Geometry check sheet. Reference: drawing and pictorial views, mm from the part's lowest x, y, z. A direction names the side the tool comes from. Coordinates: 2 decimals unless noted, no trailing zeros. Loops run counter-clockwise (first coordinate to the right, second up) from the corner with the lowest first, then second, coordinate; pieces in that order, holes last. Notation, with made-up numbers: (58.25, -16.75) - (96.25, -16.75) arc R32 ccw to (96.25, 16.25) - close; hole circle Ø9 at (-23.75, 87.5). An arc over 180 degrees is marked (long way). Use a Markdown table: item, result. Add a question column.
1) Thickness scan on line 1 (X direction, y = 1.25, z = 8.75); line 2 (X direction, y = 4, z = 1.5); line 3 (Y direction, x = 4, z = 5.75). Record the ranges inside material, lowest first.
2) Sectioned sample at B-B, the plane x = 3.66. Enter the section's corners in (y, z).
3) Sectioned sample at D-D, the plane x = 8. Enter the section's corners in (y, z), then the cut area to 3 significant figures.
4) Draft check along X on the marked faces 3, 4 and 5. Enter one of: pulls with the +X half, pulls with the -X half, needs draft (parallel to the pull), parting line crosses it, or undercut.
5) Sectioned sample at C-C, the plane y = 0.5. Enter the section's corners in (x, z).
6) Tool access check on the marked faces 1 and 2. Record the directions out of +Z, -Z, +X, -X, +Y, -Y that give a thin tool (end or side, any length) a straight path to the whole face; none if there is none.
7) Sectioned sample at A-A, the plane z = 5.5. State how many separate pieces and enclosed holes the cut face has, then the cut area to 3 significant figures.
8) Go/stop test with flat-tipped pins: P1, Ø2, axis at x = 3, z = 1, coming from the +Y side; P2, Ø1, axis at x = 9.5, y = 2, coming from the -Z side. Record where each tip stops, or that it passes through.
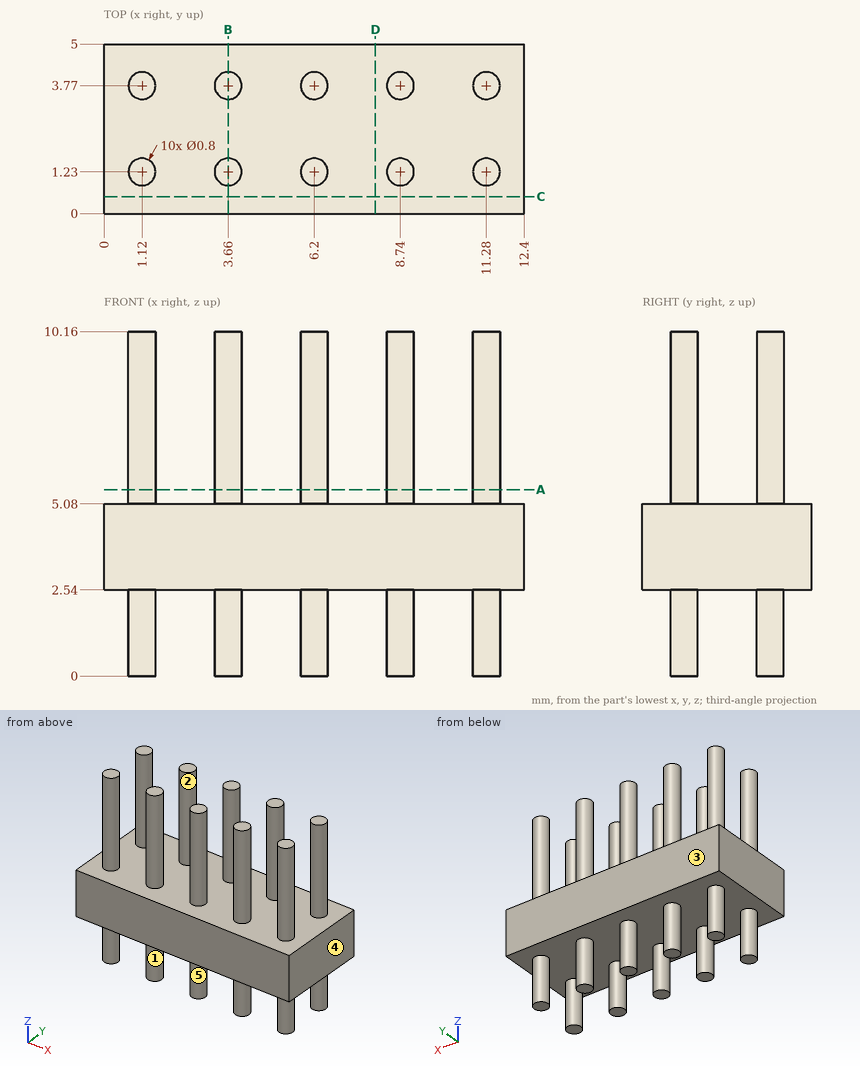
Solved:
| question | item | result |
|---|---|---|
| 1 | line 1 | x = 0.72 to 1.52, 3.26 to 4.06, 5.8 to 6.6, 8.34 to 9.14, 10.88 to 11.68 |
| 1 | line 2 | x = 0.79 to 1.45, 3.33 to 3.99, 5.87 to 6.53, 8.41 to 9.07, 10.95 to 11.61 |
| 1 | line 3 | y = 1.02 to 1.44, 3.56 to 3.98 |
| 2 | outline | (0, 2.54) - (0.83, 2.54) - (0.83, 0) - (1.63, 0) - (1.63, 2.54) - (3.37, 2.54) - (3.37, 0) - (4.17, 0) - (4.17, 2.54) - (5, 2.54) - (5, 5.08) - (4.17, 5.08) - (4.17, 10.16) - (3.37, 10.16) - (3.37, 5.08) - (1.63, 5.08) - (1.63, 10.16) - (0.83, 10.16) - (0.83, 5.08) - (0, 5.08) - close |
| 3 | outline | (0, 2.54) - (5, 2.54) - (5, 5.08) - (0, 5.08) - close |
| 3 | area | 12.7 mm2 |
| 4 | face 3 | needs draft |
| 4 | face 4 | pulls with the +X half |
| 4 | face 5 | undercut |
| 5 | outline | (0, 2.54) - (12.4, 2.54) - (12.4, 5.08) - (0, 5.08) - close |
| 6 | face 1 | -Z |
| 6 | face 2 | +Z |
| 7 | separate pieces | 10 |
| 7 | enclosed holes | 0 |
| 7 | area | 5.03 mm2 |
| 8 | P1 | stops at y = 4.17 |
| 8 | P2 | stops at z = 2.54 |
